CAD build for the part. Positions are in the model's coordinates, mm. A direction names the side the tool comes from. Coordinates: 2 decimals unless noted, no trailing zeros. Loops run counter-clockwise (first coordinate to the right, second up) from the corner with the lowest first, then second, coordinate; pieces in that order, holes last.
1) Saw through at D-D, the plane x = -45. Write the cut outline in (y, z).
2) Two-plate mould, pull along Z, no slides. Class faces 4 (the cylindrical face through (51.73, -37.33, -21.45)), 5 (the cylindrical face through (11.923, -0.986, 3.755)), 6 (the flat face through (-23, -25, 52)): +Z half, -Z half, draft (parallel to the pull), parting line (faces both ways), or undercut.
3) Which spindle directions (+Z, -Z, +X, -X, +Y, -Y) get a long thin tool onto all of the face, cutting with end or side? Do faces 1 (the cylindrical face through (49.45, -21.2, 43.28)), 2 (the cylindrical face through (51.73, -8.63, -21.45)), 3 (the flat face through (11, -2, -11)). Say none if no direction does.
4) Saw through at A-A, the plane x = 0. Write the cut outline in (y, z), and give its area (3 significant figures).
5) Pin check, flat tips, straight feed: pin 1 Ø1 at (x, y) = (-18.5, -19.5) entering from -Z; pin 2 Ø12 at (y, z) = (-35.5, 52.5) entering from -X; pin 3 Ø12 at (y, z) = (-19.5, -22.5) entering from -X. Stop position of each tip, or through.
6) Saw through at C-C, the plane y = -44. Write the cut outline in (x, z), and give its area (3 significant figures).
7) Wall check: line 1 along Z through (x, y) = (0, -1.3); line 2 along Y through (x, z) = (-25, 67.5); line 3 along Y through (x, z) = (-27, -22.5). Give the ranges that are in metal, low to high.
8) Saw through at B-B, the plane z = 0. Write the cut outline in (x, y), and give its area (3 significant figures).
```python
from build123d import *

# Parameters (mm, degrees)
F0_R     = 56
F0_R_2   = 51
F1_DEPTH = 50
F0_R_3   = 77
F2_DEPTH = 25
F3_DEPTH = 17.5
F5_D     = 8.8
F6_R     = 51
F6_R_2   = 12.5
F7_DEPTH = 2


with BuildPart() as f1:
    # F0 (on Front) → F1 (new body)
    with BuildSketch(Plane.XZ):
        Circle(F0_R)
        Circle(F0_R_2, mode=Mode.SUBTRACT)
    extrude(amount=F1_DEPTH)

    # F0 (on Front) → F2 (join)
    with BuildSketch(Plane.XZ):
        Circle(F0_R_3)
        Circle(F0_R, mode=Mode.SUBTRACT)
    extrude(amount=F2_DEPTH)

    # F0 (on Front) → F3 (cut)
    with BuildSketch(Plane.XZ):
        Circle(F0_R_3)
        Circle(F0_R, mode=Mode.SUBTRACT)
    extrude(amount=F3_DEPTH, mode=Mode.SUBTRACT)

    # F5 (through all)
    with Locations(Plane.XZ.offset(25)):
        with Locations((-45.962, 45.962), (45.9618815542, 45.962), (45.9618815542, -45.962), (-45.962, -45.962)):
            Hole(F5_D / 2)

    # F6 (on Front) → F7 (join)
    with BuildSketch(Plane.XZ):
        Circle(F6_R)
        Circle(F6_R_2, mode=Mode.SUBTRACT)
    extrude(amount=F7_DEPTH)


solid = f1.part
```
Data:
1. outline: (-50, -33.33) - (-25, -33.33) - (-25, -41.67) - (-17.5, -41.67) - (-17.5, -33.33) - (0, -33.33) - (0, 33.33) - (-17.5, 33.33) - (-17.5, 41.67) - (-25, 41.67) - (-25, 33.33) - (-50, 33.33) - (-50, 24) - (-2, 24) - (-2, -24) - (-50, -24) - close; (-25, -62.48) - (-17.5, -62.48) - (-17.5, -50.26) - (-25, -50.26) - close; (-25, 50.26) - (-17.5, 50.26) - (-17.5, 62.48) - (-25, 62.48) - close
2. face 4: parting line
2. face 5: undercut
2. face 6: draft
3. face 1: +Y, -Y
3. face 2: +Y
3. face 3: -Y
4. outline: (-50, -56) - (-25, -56) - (-25, -77) - (-17.5, -77) - (-17.5, -56) - (0, -56) - (0, -12.5) - (-2, -12.5) - (-2, -51) - (-50, -51) - close; (-50, 51) - (-2, 51) - (-2, 12.5) - (0, 12.5) - (0, 56) - (-17.5, 56) - (-17.5, 77) - (-25, 77) - (-25, 56) - (-50, 56) - close
4. area: 969 mm2
5. pin 1: stops at z = -74.87
5. pin 2: stops at x = -31.2
5. pin 3: stops at x = -75.21
6. outline: circle Ø112 at (0, 0); hole circle Ø102 at (0, 0)
6. area: 1,680 mm2
7. line 1: z = -56 to -12.5, 12.5 to 56
7. line 2: y = -25 to -17.5
7. line 3: y = -2 to 0
8. outline: (-77, -25) - (-56, -25) - (-56, -50) - (-51, -50) - (-51, -2) - (-12.5, -2) - (-12.5, 0) - (-56, 0) - (-56, -17.5) - (-77, -17.5) - close; (12.5, -2) - (51, -2) - (51, -50) - (56, -50) - (56, -25) - (77, -25) - (77, -17.5) - (56, -17.5) - (56, 0) - (12.5, 0) - close
8. area: 969 mm2
